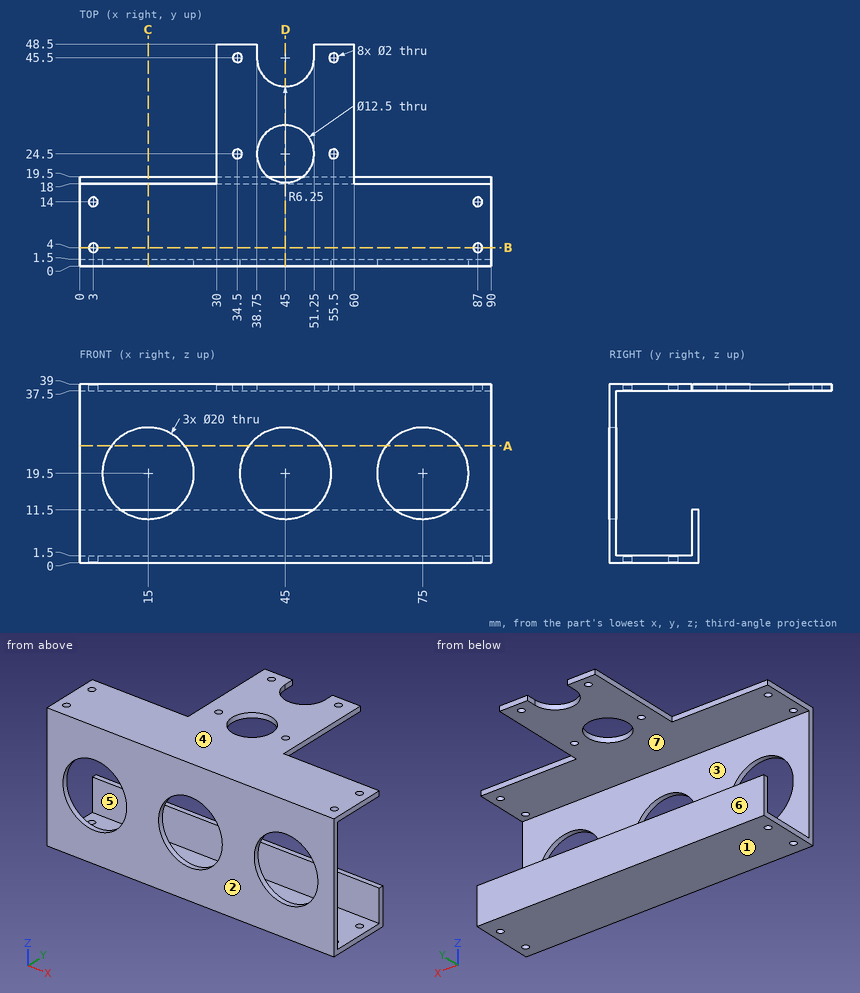
Study the drawing (mm; zero at the part's minimum x, y, z) and answer. A direction names the side the tool comes from. Round coordinates to 2 decimals unless told otherwise and drop trailing zeros. Write each loop counter-clockwise with the first axis right and the second up, starting at its lowest first coordinate (ties: lowest second). Pieces come first, ordered by that corner, then holes.
1) A cutting plane is placed at C-C (x = 15). Give the vertices of the cut face in (y, z).
2) A cutting plane is placed at D-D (x = 45). Give the vertices of the cut face in (y, z).
3) The mould has two halves that part along Z. Classify the marked faces 1, 2 and 3: pulls with the +Z half, pulls with the -Z half, needs draft (parallel to the pull), parting line crosses it, or undercut.
4) A cutting plane is placed at B-B (y = 4). Give the vertices of the cut face in (x, z), plus the area to 3 significant figures.
5) Given pin 1 Ø6 at (x, z) = (27, 4.5) entering from +Y; pin 2 Ø1.2 at (x, y) = (3, 4) entering from +Z; pin 3 Ø0.8 at (x, z) = (81.5, 38) entering from +Y; pin 4 Ø1.2 at (y, z) = (46.5, 38.5) entering from -X, each flat-ended and moving along its own axis, determine where each tip first touches the part or whether it passes through.
6) Straight lines are drawn through the part: line 1 (Y direction, x = 87, z = 0.4); line 2 (Y direction, x = 61.5, z = 6); line 3 (Z direction, x = 34.5, y = 2). For each, find the intervals that lie inside material, in ascending order.
7) A tool of negligible diameter and unlimited length cuts with its end or side. For the marked faces 4, 5, 6 and 7, from which of +Z, -Z, +X, -X, +Y, -Y can it reach the whole face along a straight path? Write none if from no direction.
8) A cutting plane is placed at A-A (z = 25.5). Give the vertices of the cut face in (x, y).
Completed:
1. outline: (0, 0) - (19.5, 0) - (19.5, 11.5) - (18, 11.5) - (18, 1.5) - (1.5, 1.5) - (1.5, 9.5) - (0, 9.5) - close; (0, 29.5) - (1.5, 29.5) - (1.5, 37.5) - (18, 37.5) - (18, 39) - (0, 39) - close
2. outline: (0, 0) - (19.5, 0) - (19.5, 11.5) - (18, 11.5) - (18, 1.5) - (1.5, 1.5) - (1.5, 9.5) - (0, 9.5) - close; (0, 29.5) - (1.5, 29.5) - (1.5, 37.5) - (18.25, 37.5) - (18.25, 39) - (0, 39) - close; (30.75, 37.5) - (39.25, 37.5) - (39.25, 39) - (30.75, 39) - close
3. face 1: pulls with the -Z half
3. face 2: needs draft
3. face 3: undercut
4. outline: (0, 0) - (2, 0) - (2, 1.5) - (0, 1.5) - close; (0, 37.5) - (2, 37.5) - (2, 39) - (0, 39) - close; (4, 0) - (86, 0) - (86, 1.5) - (4, 1.5) - close; (4, 37.5) - (86, 37.5) - (86, 39) - (4, 39) - close; (88, 0) - (90, 0) - (90, 1.5) - (88, 1.5) - close; (88, 37.5) - (90, 37.5) - (90, 39) - (88, 39) - close
4. area: 258 mm2
5. pin 1: stops at y = 19.5
5. pin 2: passes through
5. pin 3: stops at y = 18
5. pin 4: stops at x = 30
6. line 1: y = 0 to 3, 5 to 13, 15 to 19.5
6. line 2: y = 0 to 1.5, 18 to 19.5
6. line 3: z = 0 to 1.5, 37.5 to 39
7. face 4: +Z, +X, -X, +Y, -Y
7. face 5: +X, -X
7. face 6: -Z, +X, -X, +Y
7. face 7: +X, -X, +Y
8. outline: (0, 0) - (7, 0) - (7, 1.5) - (0, 1.5) - close; (23, 0) - (37, 0) - (37, 1.5) - (23, 1.5) - close; (53, 0) - (67, 0) - (67, 1.5) - (53, 1.5) - close; (83, 0) - (90, 0) - (90, 1.5) - (83, 1.5) - close
